Autodesk Inventor part; units mm, degrees
ref_plane "YZ Plane" through (0, 0, 0) normal (1, 0, 0) x (0, 1, 0)
ref_plane "XZ Plane" through (0, 0, 0) normal (0, 1, 0) x (-1, 0, 0)
ref_plane "XY Plane" through (0, 0, 0) normal (0, 0, 1) x (1, 0, 0)
sketch "Sketch2" plane through (0, 0, 0) normal (1, 0, 0) x (0, 1, 0)
  circle A0 centre (0, 0) radius 1.75
extrude "Extrusion1" add sketch "Sketch2" along normal mid plane 10.2
chamfer "Chamfer1" distance 0.2 angle 45 1 edges at (5.1, -1.75, 0) measured on face at (5.1, -0.5165, 0.5026)
sketch "Sketch3" plane through (-5.1, 0, 0) normal (-1, 0, 0) x (0, 0, 1)
  circle A0 centre (0, 0) radius 1.75
  dimension "d27" = 3.5
extrude "Extrusion2" add sketch "Sketch3" along normal blind 0.32
chamfer "Chamfer2" distance 0.32 angle 45 1 edges at (-5.42, 0, -1.75) measured on face at (-5.42, 0.5026, -0.5165)
sketch "Sketch4" plane through (-5.42, 0, 0) normal (-1, 0, 0) x (0, 0, 1)
  circle A0 centre (0, 0) radius 1.25
  dimension "d33" = 2.5
extrude "Extrusion3" add sketch "Sketch4" along normal blind 0.41
sketch "Sketch5" plane through (0, 0, 0) normal (0, 1, 0) x (-1, 0, 0)
  line L0 (5.83, 0) -> (5.83, -1.25)
  line L1 (8.63, -2.91) -> (8.21, -2.91)
  line L2 (8.21, -2.91) -> (5.83, -1.25)
  line L3 (8.63, -2.91) -> (8.63, 0)
  line L4 (5.83, -1.25) -> (5.83, 0)
  line L5 (8.63, 0) -> (5.83, 0)
  point P0 (0, 0)
  dimension "d40" = 0.42
revolve "Revolution1" add sketch "Sketch5" angle 360 about axis through (-8.63, 0, 0) along (1, 0, 0)
sketch "Sketch6" plane through (-8.63, 0, 0) normal (-1, 0, 0) x (0, 0, 1)
  circle A0 centre (0, 0) radius 2.91
  line L0 (0.425, 2.91) -> (0.425, -2.91)
  line L1 (-0.425, 2.91) -> (-0.425, -2.91)
  line L2 (-0.425, 2.91) -> (0.425, 2.91)
  line L3 (-0.425, -2.91) -> (0.425, -2.91)
  line L4 (-0.425, 2.91) -> (0.425, 2.91)
  line L5 (0.425, 2.91) -> (0.425, -2.91)
  line L6 (0.425, -2.91) -> (-0.425, -2.91)
  line L7 (-0.425, -2.91) -> (-0.425, 2.91)
extrude "Extrusion4" cut sketch "Sketch6" against normal blind 0.5 contours L0 A0 L1 | A0 L2 L0 | L0 L3 A0 | A0 L1 L2 | L3 L1 A0
thread "Thread1"
properties part number "parafuso escariado M3,5"
Geometry check sheet. Reference: the model listing, model coordinates, mm. A direction names the side the tool comes from. Coordinates: 2 decimals unless noted, no trailing zeros. Order: outer loops, then holes, each group sorted by start corner. A loop starts at its lowest first (then second) coordinate and runs counter-clockwise, first axis right, second up. Notation, with made-up numbers: (-11, 6) - (14, 6) arc R35 cw to (14, 45) - close; hole circle Ø1 at (35, -35.5). An arc over 180 degrees is marked (long way). Answer as a JSON object with one key per item and string values. Group by question number.
Item 1: Tool access check on faces 1 (the face through (-5.98, 0.52, -1.25)), 2 (the face through (-8.63, 0, -1)). Record the directions out of +Z, -Z, +X, -X, +Y, -Y that give a thin tool (end or side, any length) a straight path to the whole face; none if there is none.
Item 2: Sectioned sample at D-D, the plane x = -6. Record the cut outline in (y, z).
Item 3: Depth check by flat-ended pin: pin 1 Ø1 at (x, y) = (-7, 0) entering from +Z. Enter the tip coordinate at first touch or a pass-through.
Item 4: Sectioned sample at C-C, the plane x = -2. Record the cut outline in (y, z).
Item 5: Draft check along X on faces 3 (the face through (-5.62, 1.22, -0.27)), 4 (the face through (5.1, 0, 0)), 5 (the face through (-8.13, 0, 0)), 6 (the face through (-8.42, 0.06, 2.91)). Enter one of: +X half, -X half, draft (parallel to the pull), parting line (faces both ways), or undercut.
Item 6: Sectioned sample at B-B, the plane z = 0. Record the cut outline in (x, y), and give its area (3 significant figures).
Item 7: Scan lines: probe 1 along Y at (x, z) = (4, 1.15); probe 2 along X at (y, z) = (2, -1.15); probe 3 along Y at (x, z) = (4, 1.4). Record each from-to range of solid material in increasing order.
Resolved:
{
 "1": {"face 1": "none", "face 2": "+Z, -Z, -X, +Y, -Y"},
 "2": {"outline": "circle Ø2.74 at (0, 0)"},
 "3": {"pin 1": "z = 2.41"},
 "4": {"outline": "circle Ø3.5 at (0, 0)"},
 "5": {"face 3": "undercut", "face 4": "+X half", "face 5": "-X half", "face 6": "draft"},
 "6": {"outline": "(-8.13, -2.85) - (-5.83, -1.25) - (-5.42, -1.25) - (-5.42, -1.43) - (-5.1, -1.75) - (4.9, -1.75) - (5.1, -1.55) - (5.1, 1.55) - (4.9, 1.75) - (-5.1, 1.75) - (-5.42, 1.43) - (-5.42, 1.25) - (-5.83, 1.25) - (-8.13, 2.85) - close", "area": "47.1 mm^2"},
 "7": {"probe 1": "-1.32 to 1.32", "probe 2": "-8.63 to -7.35", "probe 3": "-1.05 to 1.05"}
}
